```python
from build123d import *

# Parameters (mm, degrees)
SKETCH1_W           = 100
SKETCH1_H           = 254
BOSS_EXTRUDE1_DEPTH = 3
SKETCH2_W           = 50
SKETCH2_H           = 3
BOSS_EXTRUDE2_DEPTH = 3
SKETCH3_W           = 3
SKETCH3_H           = 35
SKETCH3_H_2         = 40
BOSS_EXTRUDE3_DEPTH = 3
SKETCH4_R           = 4.2
SKETCH4_R_2         = 21.25
SKETCH4_R_3         = 2.9
CUT_EXTRUDE1_DEPTH  = 3
SKETCH5_W           = 3
SKETCH5_H           = 36
SKETCH5_H_2         = 40
BOSS_EXTRUDE4_DEPTH = 3


with BuildPart() as part:
    # Sketch1 → Boss-Extrude1 (new body)
    with BuildSketch(Plane.XY):
        Rectangle(SKETCH1_W, SKETCH1_H)
    extrude(amount=BOSS_EXTRUDE1_DEPTH)

    # Sketch2 → Boss-Extrude2 (add)
    with BuildSketch(Plane.XZ.offset(127)):
        with Locations((0, 1.5)):
            Rectangle(SKETCH2_W, SKETCH2_H)
    extrude(amount=BOSS_EXTRUDE2_DEPTH)

    # Sketch3 → Boss-Extrude3 (add)
    with BuildSketch(Plane(origin=(50, 0, 0), x_dir=(0, 0, -1), z_dir=(1, 0, 0))):
        with Locations((-1.5, 72.5)):
            Rectangle(SKETCH3_W, SKETCH3_H)
        with Locations((-1.5, 0)):
            Rectangle(SKETCH3_W, SKETCH3_H_2)
        with Locations((-1.5, -72.5)):
            Rectangle(SKETCH3_W, SKETCH3_H)
    extrude(amount=BOSS_EXTRUDE3_DEPTH)

    # Sketch4 → Cut-Extrude1 (cut)
    with BuildSketch(Plane(origin=(0, 0, 0), x_dir=(-1, 0, 0), z_dir=(0, 0, -1))):
        with Locations((14, 112.8)):
            Circle(SKETCH4_R)
        with Locations((14, 70.8)):
            Circle(SKETCH4_R_2)
        with Locations((14, 28.8)):
            Circle(SKETCH4_R)
        with Locations((-16, -37)):
            Circle(SKETCH4_R_3)
        with Locations((36, -37)):
            Circle(SKETCH4_R_3)
        with Locations((36, -91)):
            Circle(SKETCH4_R_3)
        with Locations((-16, -91)):
            Circle(SKETCH4_R_3)
        with BuildLine():
            Line((9.083005244, -68.5), (10.916994756, -68.5))
            ThreePointArc((10.916994756, -68.5), (32.581133525, -67.075464159), (14.75, -54.689387775))
            Line((14.75, -54.689387775), (14.75, -49.3))
            Line((14.75, -49.3), (10, -49.3))
            Line((10, -49.3), (5.25, -49.3))
            Line((5.25, -49.3), (5.25, -54.689387775))
            ThreePointArc((5.25, -54.689387775), (-12.581133525, -67.075464159), (9.083005244, -68.5))
        make_face()
    extrude(amount=-CUT_EXTRUDE1_DEPTH, mode=Mode.SUBTRACT)

    # Sketch5 → Boss-Extrude4 (add)
    with BuildSketch(Plane.ZY.offset(50)):
        with Locations((1.5, -61)):
            Rectangle(SKETCH5_W, SKETCH5_H)
        with Locations((1.5, 17)):
            Rectangle(SKETCH5_W, SKETCH5_H_2)
        with Locations((1.5, 97)):
            Rectangle(SKETCH5_W, SKETCH5_H_2)
    extrude(amount=BOSS_EXTRUDE4_DEPTH)


solid = part.part
```
Can you work these out from the model? Positions are in its coordinate system, mm. Round coordinates to 2 decimals unless told otherwise and drop trailing zeros. Loops run counter-clockwise (first coordinate to the right, second up) from the corner with the lowest first, then second, coordinate; pieces in that order, holes last. Notation, with made-up numbers: M -15,48.5 L 13,48.5 A20 ccw 13,69.5 Z; hole C 77.25,60 d3. An arc over 180 degrees is marked long. Answer as a JSON object with one key per item and string values. Group by question number.
Q1. Imagine slicing it at D-D, the plane x = 2.5. Please give me the cut outline in (y, z).
Q2. Please list where these lines run through material, in increasing order: L1, parallel to Y at x = -36, z = 1.5; L2, parallel to Y at x = 16, z = 2.25; L3, parallel to Y at x = -14, z = 1.5.
Q3. We'd pull the mould along X, two halves only. Please class faces 1 (the cylindrical face through (-38.68, -92.11, 1.48)), 2 (the cylindrical face through (18.301, -38.765, 1.479)), 3 (the flat face through (-1, 0, 0)): +X half, -X half, draft (parallel to the pull), parting line (faces both ways), or undercut.
Q4. Imagine slicing it at C-C, the plane y = -64. Please give me the cut outline in (x, z).
Q5. Imagine slicing it at A-A, the plane x = 16. Please give me the cut outline in (y, z), then the cut area to 3 significant figures.
Q6. Will these pins go through, and if not, where does the flat tip stop? pin 1 (0.9 mm diameter, centred on x = -51, z = 1.5, fed in from -Y); pin 2 (1.5 mm diameter, centred on x = -34, z = 2, fed in from -Y); pin 3 (1.5 mm diameter, centred on x = 51, z = 1, fed in from +Y).
Q7. Imagine slicing it at B-B, the plane y = 70.8. Please give me the cut outline in (x, z).
Findings:
{
 "1": {"outline": "M -130,0 L -75.46,0 L -75.46,3 L -130,3 Z; M -52.54,0 L 57.41,0 L 57.41,3 L -52.54,3 Z; M 84.19,0 L 127,0 L 127,3 L 84.19,3 Z"},
 "2": {"L1": "y = -127 to -93.9, -88.1 to -39.9, -34.1 to 127", "L2": "y = -130 to -93.9, -88.1 to -39.9, -34.1 to 127", "L3": "y = -130 to -72.72, -49.3 to 24.6, 33 to 49.55, 92.05 to 108.6, 117 to 127"},
 "3": {"face 1": "undercut", "face 2": "undercut", "face 3": "draft"},
 "4": {"outline": "M -53,0 L -33,0 L -33,3 L -53,3 Z; M 13,0 L 53,0 L 53,3 L 13,3 Z"},
 "5": {"outline": "M -130,0 L -93.9,0 L -93.9,3 L -130,3 Z; M -88.1,0 L -39.9,0 L -39.9,3 L -88.1,3 Z; M -34.1,0 L 127,0 L 127,3 L -34.1,3 Z", "area": "736 mm2"},
 "6": {"pin 1": "stops at y = -79", "pin 2": "stops at y = -127", "pin 3": "stops at y = 90"},
 "7": {"outline": "M -50,0 L -35.25,0 L -35.25,3 L -50,3 Z; M 7.25,0 L 53,0 L 53,3 L 7.25,3 Z"}
}
